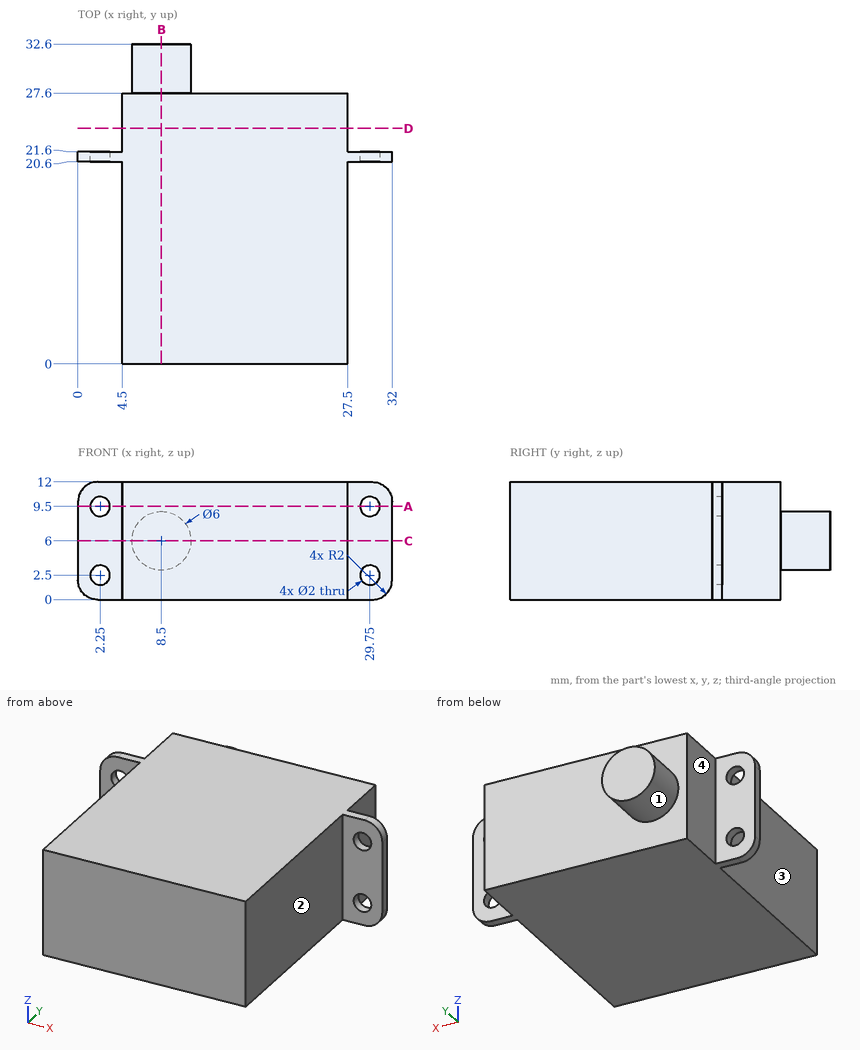
Part print with two shaded views. Sizes in mm from the minimum x, y, z corner. A direction names the side the tool comes from. Round coordinates to 2 decimals unless told otherwise and drop trailing zeros. Order: outer loops, then holes, each group sorted by start corner. A loop starts at its lowest first (then second) coordinate and runs counter-clockwise, first axis right, second up. Notation, with made-up numbers: (1, 73.5) - (11, 73.5) arc R21 cw to (11, 106.5) - close; hole circle Ø11 at (76, 1.5). An arc over 180 degrees is marked (long way). Answer in a Markdown table with one row per item. Add a question column.
(1) Probe L1, parallel to X at y = 21.35, z = 2.5; L2, parallel to Z at x = 29.75, y = 21; L3, parallel to Z at x = 29, y = 21. List the from-to ranges inside material, lowest first. Write a range as [from, to].
(2) Band-saw the part on D-D on y = 24. List the corners of the cut face in (x, z), and give its area (3 significant figures).
(3) Band-saw the part on A-A on z = 9.5. List the corners of the cut face in (x, y), and give its area (3 significant figures).
(4) Drop flat-ended pins along their axis: pin 1 Ø6 at (y, z) = (27.5, 8.5) entering from +X; pin 2 Ø6 at (y, z) = (13, 4) entering from -X; pin 3 Ø1.3 at (x, z) = (2.5, 4.5) entering from -Y; pin 4 Ø1.2 at (x, z) = (2.25, 9.5) entering from -Y. Give the stop position or say it passes through.
(5) Band-saw the part on B-B on x = 8.5. List the corners of the cut face in (y, z).
(6) 3-axis set-ups, long thin cutter, end or side, ignore diameter. For the marked faces 1, 2, 3 and 4: which of +Z, -Z, +X, -X, +Y, -Y reach the whole face in a straight line?
(7) Band-saw the part on C-C on z = 6. List the corners of the cut face in (x, y).
Data:
| question | item | result |
|---|---|---|
| 1 | L1 | x = [0, 1.25], [3.25, 28.75], [30.75, 32] |
| 1 | L2 | z = [0, 1.5], [3.5, 8.5], [10.5, 12] |
| 1 | L3 | z = [0, 1.84], [3.16, 8.84], [10.16, 12] |
| 2 | outline | (4.5, 0) - (27.5, 0) - (27.5, 12) - (4.5, 12) - close |
| 2 | area | 276 mm^2 |
| 3 | outline | (0, 20.6) - (1.25, 20.6) - (1.25, 21.6) - (0, 21.6) - close; (3.25, 20.6) - (4.5, 20.6) - (4.5, 0) - (27.5, 0) - (27.5, 20.6) - (28.75, 20.6) - (28.75, 21.6) - (27.5, 21.6) - (27.5, 27.6) - (4.5, 27.6) - (4.5, 21.6) - (3.25, 21.6) - close; (30.75, 20.6) - (32, 20.6) - (32, 21.6) - (30.75, 21.6) - close |
| 3 | area | 640 mm^2 |
| 4 | pin 1 | stops at x = 27.5 |
| 4 | pin 2 | stops at x = 4.5 |
| 4 | pin 3 | stops at y = 20.6 |
| 4 | pin 4 | passes through |
| 5 | outline | (0, 0) - (27.6, 0) - (27.6, 3) - (32.6, 3) - (32.6, 9) - (27.6, 9) - (27.6, 12) - (0, 12) - close |
| 6 | face 1 | +Y |
| 6 | face 2 | +Z, -Z, +X, -Y |
| 6 | face 3 | +Z, -Z, -X, -Y |
| 6 | face 4 | +Z, -Z, -X, +Y |
| 7 | outline | (0, 20.6) - (4.5, 20.6) - (4.5, 0) - (27.5, 0) - (27.5, 20.6) - (32, 20.6) - (32, 21.6) - (27.5, 21.6) - (27.5, 27.6) - (11.5, 27.6) - (11.5, 32.6) - (5.5, 32.6) - (5.5, 27.6) - (4.5, 27.6) - (4.5, 21.6) - (0, 21.6) - close |
